CAD build for the part. Positions are in the model's coordinates, mm. Give positions to 0.01 mm unless a question says otherwise; leave off trailing zeros. Write each loop counter-clockwise with the first axis right and the second up, starting at its lowest first coordinate (ties: lowest second). Pieces come first, ordered by that corner, then holes. Notation, with made-up numbers: (-23, -38) -> (26, -38) arc R22 cw to (26, -31) -> close; hole circle Ø5 at (28.25, -14.75). An arc over 180 degrees is marked (long way). Answer as a JSON object with one key per item and string values.
```python
from build123d import *

# Parameters (mm, degrees)
SKETCH_1_R      = 3.25
SKETCH_1_R_2    = 0.6
EXTRUDE_1_DEPTH = 0.35


with BuildPart() as part:
    # Эскиз1 → Вытянуть1 (new body)
    with BuildSketch(Plane.XY):
        with BuildLine():
            Line((2.380261504, 4.86702901), (1.731990268, 9.350710913))
            ThreePointArc((1.731990268, 9.350710913), (0, 10.850291839), (-1.731990268, 9.350710913))
            Line((-1.731990268, 9.350710913), (-2.380261504, 4.86702901))
            ThreePointArc((-2.380261504, 4.86702901), (-2.610401545, 4.183671542), (-3.067922226, 3.626341575))
            ThreePointArc((-3.067922226, 3.626341575), (0, -4.75), (3.067922226, 3.626341575))
            ThreePointArc((3.067922226, 3.626341575), (2.610401545, 4.183671542), (2.380261504, 4.86702901))
        make_face()
        Circle(SKETCH_1_R, mode=Mode.SUBTRACT)
        with Locations((0, 9.100291839)):
            Circle(SKETCH_1_R_2, mode=Mode.SUBTRACT)
    extrude(amount=EXTRUDE_1_DEPTH)


solid = part.part
```
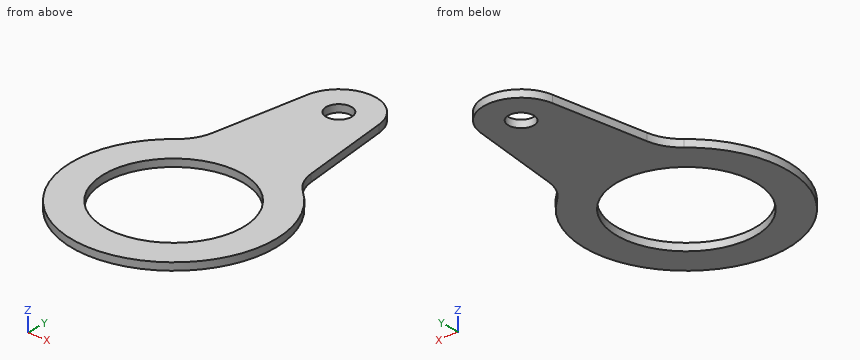
1) Slice it at C-C (z = 0.25). List the corners of the cut face in (x, y), then the cut area to 3 significant figures.
Model answer:
{"outline": "(-3.07, 3.63) arc R4.75 ccw (long way) to (3.07, 3.63) arc R2 cw to (2.38, 4.87) -> (1.73, 9.35) arc R1.75 ccw to (-1.73, 9.35) -> (-2.38, 4.87) arc R2 cw to start; hole circle Ø6.5 at (0, 0); hole circle Ø1.2 at (0, 9.1)", "area": "60.7 mm2"}
2) Slice it at B-B (y = 0). List the corners of the cut face in (x, z).
Model answer:
{"outline": "(-4.75, 0) -> (-3.25, 0) -> (-3.25, 0.35) -> (-4.75, 0.35) -> close; (3.25, 0) -> (4.75, 0) -> (4.75, 0.35) -> (3.25, 0.35) -> close"}
3) Wall check: probe 1 along Y at (x, z) = (-1, 0.1); probe 2 along Y at (x, z) = (1.25, 0.2); probe 3 along X at (y, z) = (0.25, 0.2). Give the ranges that are in metal, low to high.
Model answer:
{"probe 1": "y = -4.64 to -3.09, 3.09 to 10.54", "probe 2": "y = -4.58 to -3, 3 to 10.33", "probe 3": "x = -4.74 to -3.24, 3.24 to 4.74"}
4) Slice it at A-A (x = 0). List the corners of the cut face in (y, z), then the cut area to 3 significant figures.
Model answer:
{"outline": "(-4.75, 0) -> (-3.25, 0) -> (-3.25, 0.35) -> (-4.75, 0.35) -> close; (3.25, 0) -> (8.5, 0) -> (8.5, 0.35) -> (3.25, 0.35) -> close; (9.7, 0) -> (10.85, 0) -> (10.85, 0.35) -> (9.7, 0.35) -> close", "area": "2.77 mm2"}
5) Pin check, flat tip, straight feed: pin 1 (1.6 mm diameter, centred on x = 0, y = 9.1, fed in from -Z). Stop position of the tip, or through.
Model answer:
{"pin 1": "stops at z = 0"}
6) Slice it at D-D (y = 2). List the corners of the cut face in (x, z), then the cut area to 3 significant figures.
Model answer:
{"outline": "(-4.31, 0) -> (-2.56, 0) -> (-2.56, 0.35) -> (-4.31, 0.35) -> close; (2.56, 0) -> (4.31, 0) -> (4.31, 0.35) -> (2.56, 0.35) -> close", "area": "1.22 mm2"}
